Part model, mm, in its own coordinate system. Face numbers are marked on the shaded views. A direction names the side the tool comes from. Round coordinates to 2 decimals unless told otherwise and drop trailing zeros. Write each loop counter-clockwise with the first axis right and the second up, starting at its lowest first coordinate (ties: lowest second). Pieces come first, ordered by that corner, then holes.
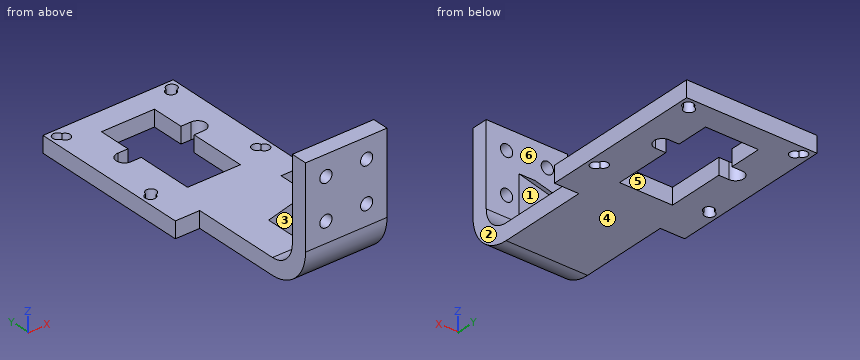
```python
from build123d import *

# Parameters (mm, degrees)
EXTRUDE_1_DEPTH     = 4
EXTRUDE_3_DEPTH     = 20
RIB_1_REACH         = 70.964
SKETCH_5_WALL_W     = 163.463051102
SKETCH_5_WALL_H     = 4
SKETCH_6_R          = 1.5
CUT_EXTRUDE_3_DEPTH = 10


with BuildPart() as part:
    # 草图1 → 凸台-拉伸1 (new body)
    with BuildSketch(Plane.XY):
        Polygon((0, 20), (0, 0), (20, 0), (20, 20), (26, 20), (26, 60), (-6, 60), (-6, 20), align=None)
        with BuildLine():
            Line((3.5, 54), (3.5, 46))
            Line((3.5, 46), (1, 46))
            ThreePointArc((1, 46), (-1, 44), (1, 42))
            Line((1, 42), (3.5, 42))
            Line((3.5, 42), (3.5, 28))
            Line((3.5, 28), (16.5, 28))
            Line((16.5, 28), (16.5, 42))
            Line((16.5, 42), (19, 42))
            ThreePointArc((19, 42), (21, 44), (19, 46))
            Line((19, 46), (16.5, 46))
            Line((16.5, 46), (16.5, 54))
            Line((16.5, 54), (3.5, 54))
        make_face(mode=Mode.SUBTRACT)
        with BuildLine():
            ThreePointArc((24.228868987, 56.771131013), (24.883883476, 58.883883476), (22.771131013, 58.228868987))
            ThreePointArc((22.771131013, 58.228868987), (22.116116524, 56.116116524), (24.228868987, 56.771131013))
        make_face(mode=Mode.SUBTRACT)
        with BuildLine():
            ThreePointArc((24.228868987, 31.228868987), (22.116116524, 31.883883476), (22.771131013, 29.771131013))
            ThreePointArc((22.771131013, 29.771131013), (24.883883476, 29.116116524), (24.228868987, 31.228868987))
        make_face(mode=Mode.SUBTRACT)
        with BuildLine():
            ThreePointArc((-4.228868987, 31.228868987), (-4.883883476, 29.116116524), (-2.771131013, 29.771131013))
            ThreePointArc((-2.771131013, 29.771131013), (-2.116116524, 31.883883476), (-4.228868987, 31.228868987))
        make_face(mode=Mode.SUBTRACT)
        with BuildLine():
            ThreePointArc((-2.771131013, 58.228868987), (-4.883883476, 58.883883476), (-4.228868987, 56.771131013))
            ThreePointArc((-4.228868987, 56.771131013), (-2.116116524, 56.116116524), (-2.771131013, 58.228868987))
        make_face(mode=Mode.SUBTRACT)
    extrude(amount=EXTRUDE_1_DEPTH)

    # 草图4 → 凸台-拉伸3 (add)
    with BuildSketch(Plane.ZY):
        with BuildLine():
            Line((0, 0), (0, -2))
            ThreePointArc((0, -2), (2.928932188, -9.071067812), (10, -12))
            Line((10, -12), (30, -12))
            Line((30, -12), (30, -8))
            Line((30, -8), (10, -8))
            ThreePointArc((10, -8), (5.757359313, -6.242640687), (4, -2))
            Line((4, -2), (4, 0))
            Line((4, 0), (0, 0))
        make_face()
    extrude(amount=-EXTRUDE_3_DEPTH)

    # 草图5 wall → 筋1 (add, up to next)
    with BuildSketch(Plane(origin=(10, 0.678932188, 12.321067812), x_dir=(0, 0.707106781187, -0.707106781187), z_dir=(0, -0.707106781187, -0.707106781187)), mode=Mode.PRIVATE) as rib_1_sk1:
        Rectangle(SKETCH_5_WALL_W, SKETCH_5_WALL_H)
    rib_1_tool1 = extrude(rib_1_sk1.sketch, amount=RIB_1_REACH, mode=Mode.PRIVATE) - part.part
    add(rib_1_tool1.solids().sort_by_distance((10, 0.678932188, 12.321067812))[0])

    # 草图6 → 切除-拉伸3 (cut)
    with BuildSketch(Plane.XZ.offset(12)):
        with Locations((5, 25)):
            Circle(SKETCH_6_R)
        with Locations((5, 15)):
            Circle(SKETCH_6_R)
        with Locations(Location((15, 15, 0), (0, 0, 90))):
            Circle(SKETCH_6_R)
        with Locations(Location((15, 25, 0), (0, 0, 90))):
            Circle(SKETCH_6_R)
    extrude(amount=-CUT_EXTRUDE_3_DEPTH, mode=Mode.SUBTRACT)


solid = part.part
```
Q1. Mould opens along Y. For the marked faces 4, 5 and 6 say: +Y half, -Y half, draft (parallel to the pull), parting line (faces both ways), or undercut.
Values follow:
face 4: draft
face 5: undercut
face 6: +Y half
Q2. Cut at C-C on x = 15. Write the cut outline in (y, z), plus the area to 3 significant figures.
Values follow:
outline: (-12, 10) arc R10 ccw to (-2, 0) - (28, 0) - (28, 4) - (-2, 4) arc R6 cw to (-8, 10) - (-8, 13.5) - (-12, 13.5) - close; (-12, 16.5) - (-8, 16.5) - (-8, 23.5) - (-12, 23.5) - close; (-12, 26.5) - (-8, 26.5) - (-8, 30) - (-12, 30) - close; (54, 0) - (60, 0) - (60, 4) - (54, 4) - close
area: 250 mm2
Q3. Cut at B-B on y = 44. Write the cut outline in (x, z).
Values follow:
outline: (-6, 0) - (-1, 0) - (-1, 4) - (-6, 4) - close; (21, 0) - (26, 0) - (26, 4) - (21, 4) - close
Q4. Which spindle directions (+Z, -Z, +X, -X, +Y, -Y) get a long thin tool onto all of the face, cutting with end or side? Do the marked faces 1, 2 and 3. Say none if no direction does.
Values follow:
face 1: +Z, +X, +Y
face 2: +Z, -Z, +X, -Y
face 3: +Z, -X, +Y
Q5. Cut at A-A on z = 25. Write the cut outline in (x, y).
Values follow:
outline: (0, -12) - (3.5, -12) - (3.5, -8) - (0, -8) - close; (6.5, -12) - (13.5, -12) - (13.5, -8) - (6.5, -8) - close; (16.5, -12) - (20, -12) - (20, -8) - (16.5, -8) - close
Q6. Wall check: L1, parallel to X at y = 58, z = 2.8; L2, parallel to Y at x = -4, z = 2.4; L3, parallel to Z at x = 5.5, y = 54.5. Give the ranges that are in metal, low to high.
Values follow:
L1: x = -6 to -5.25, -2.25 to 22.25, 25.25 to 26
L2: y = 20 to 28.75, 31.75 to 56.25, 59.25 to 60
L3: z = 0 to 4
Q7. Cut at D-D on x = 11. Write the cut outline in (y, z).
Values follow:
outline: (-12, 10) arc R10 ccw to (-2, 0) - (28, 0) - (28, 4) - (9, 4) - (-8, 21) - (-8, 30) - (-12, 30) - close; (54, 0) - (60, 0) - (60, 4) - (54, 4) - close
Q8. Drop flat-ended pins along their axis: pin 1 (0.8 mm diameter, centred on x = 17, z = 2.5, fed in from -Y); pin 2 (1.2 mm diameter, centred on x = 23, z = 3, fed in from -Y); pin 3 (10 mm diameter, centred on x = 16, z = 22, fed in from +Y). Give the stop position or say it passes through.
Values follow:
pin 1: stops at y = -9.04
pin 2: stops at y = 20
pin 3: stops at y = -6
